The listing builds one solid part. Answer for the finished solid, in the listing's coordinates (mm). Give positions to 0.01 mm unless a question says otherwise; leave off trailing zeros. Order: outer loops, then holes, each group sorted by start corner. A loop starts at its lowest first (then second) coordinate and runs counter-clockwise, first axis right, second up. Notation, with made-up numbers: (34, 47.5) - (58, 47.5) arc R16 cw to (58, 64.5) - close; hole circle Ø3 at (-1.75, -39). An arc over 180 degrees is marked (long way). Answer in a Markdown table with one row per item.
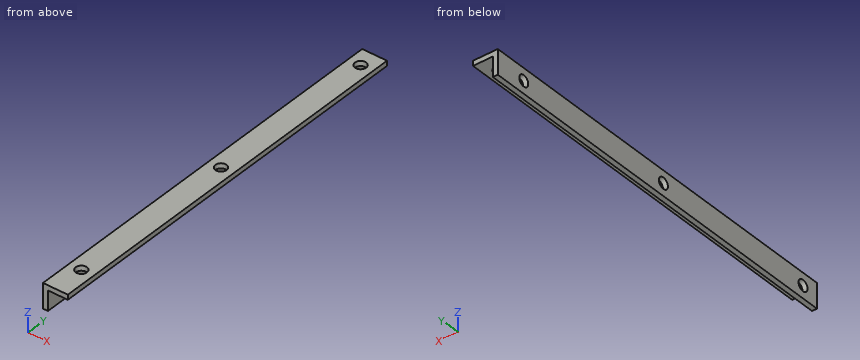
from build123d import *

# Parameters (mm, degrees)
EXTRUDE_1_DEPTH     = 160
CUT_EXTRUDE_1_REACH = 12
SKETCH_2_R          = 2.25
CUT_EXTRUDE_2_REACH = 12
SKETCH_3_R          = 2.25


with BuildPart() as part:
    # Эскиз1 → Бобышка-Вытянуть1 (new body)
    with BuildSketch(Plane(origin=(0, 0, 0), x_dir=(1, 0, 0), z_dir=(0, 1, 0))):
        Polygon((0, 10), (0, 0), (10, 0), (10, 2), (2, 2), (2, 10), align=None)
    extrude(amount=EXTRUDE_1_DEPTH)

    # Эскиз2 → Вырез-Вытянуть1 (cut, up to next)
    with BuildSketch(Plane.XY, mode=Mode.PRIVATE) as cut_extrude_1_sk1:
        with Locations((5, 13)):
            Circle(SKETCH_2_R)
    cut_extrude_1_tool1 = extrude(cut_extrude_1_sk1.sketch, amount=-CUT_EXTRUDE_1_REACH, mode=Mode.PRIVATE) & part.part
    add(cut_extrude_1_tool1.solids().sort_by_distance((5, 13, 0))[0], mode=Mode.SUBTRACT)
    # Эскиз2 → Вырез-Вытянуть1 (cut, up to next)
    with BuildSketch(Plane.XY, mode=Mode.PRIVATE) as cut_extrude_1_sk2:
        with Locations((5, 83)):
            Circle(SKETCH_2_R)
    cut_extrude_1_tool2 = extrude(cut_extrude_1_sk2.sketch, amount=-CUT_EXTRUDE_1_REACH, mode=Mode.PRIVATE) & part.part
    add(cut_extrude_1_tool2.solids().sort_by_distance((5, 83, 0))[0], mode=Mode.SUBTRACT)
    # Эскиз2 → Вырез-Вытянуть1 (cut, up to next)
    with BuildSketch(Plane.XY, mode=Mode.PRIVATE) as cut_extrude_1_sk3:
        with Locations((5, 153)):
            Circle(SKETCH_2_R)
    cut_extrude_1_tool3 = extrude(cut_extrude_1_sk3.sketch, amount=-CUT_EXTRUDE_1_REACH, mode=Mode.PRIVATE) & part.part
    add(cut_extrude_1_tool3.solids().sort_by_distance((5, 153, 0))[0], mode=Mode.SUBTRACT)

    # Эскиз3 → Вырез-Вытянуть2 (cut, up to next)
    with BuildSketch(Plane.ZY, mode=Mode.PRIVATE) as cut_extrude_2_sk1:
        with Locations((-5, 7)):
            Circle(SKETCH_3_R)
    cut_extrude_2_tool1 = extrude(cut_extrude_2_sk1.sketch, amount=-CUT_EXTRUDE_2_REACH, mode=Mode.PRIVATE) & part.part
    add(cut_extrude_2_tool1.solids().sort_by_distance((0, 7, -5))[0], mode=Mode.SUBTRACT)
    # Эскиз3 → Вырез-Вытянуть2 (cut, up to next)
    with BuildSketch(Plane.ZY, mode=Mode.PRIVATE) as cut_extrude_2_sk2:
        with Locations((-5, 77)):
            Circle(SKETCH_3_R)
    cut_extrude_2_tool2 = extrude(cut_extrude_2_sk2.sketch, amount=-CUT_EXTRUDE_2_REACH, mode=Mode.PRIVATE) & part.part
    add(cut_extrude_2_tool2.solids().sort_by_distance((0, 77, -5))[0], mode=Mode.SUBTRACT)
    # Эскиз3 → Вырез-Вытянуть2 (cut, up to next)
    with BuildSketch(Plane.ZY, mode=Mode.PRIVATE) as cut_extrude_2_sk3:
        with Locations((-5, 147)):
            Circle(SKETCH_3_R)
    cut_extrude_2_tool3 = extrude(cut_extrude_2_sk3.sketch, amount=-CUT_EXTRUDE_2_REACH, mode=Mode.PRIVATE) & part.part
    add(cut_extrude_2_tool3.solids().sort_by_distance((0, 147, -5))[0], mode=Mode.SUBTRACT)


solid = part.part
Item 1: Find section B-B on y = 153. Write down the section's boundary in (x, z), then the cut area to 3 significant figures.
Answer block:
| item | result |
|---|---|
| outline | (0, -10) - (2, -10) - (2, -2) - (2.75, -2) - (2.75, 0) - (0, 0) - close; (7.25, -2) - (10, -2) - (10, 0) - (7.25, 0) - close |
| area | 27.0 mm² |
Item 2: Find section C-C on y = 126.5. Write down the section's boundary in (x, z), then the cut area to 3 significant figures.
Answer block:
| item | result |
|---|---|
| outline | (0, -10) - (2, -10) - (2, -2) - (10, -2) - (10, 0) - (0, 0) - close |
| area | 36.0 mm² |
Item 3: Find section A-A on z = -5. Write down the section's boundary in (x, y).
Answer block:
| item | result |
|---|---|
| outline | (0, 0) - (2, 0) - (2, 4.75) - (0, 4.75) - close; (0, 9.25) - (2, 9.25) - (2, 74.75) - (0, 74.75) - close; (0, 79.25) - (2, 79.25) - (2, 144.75) - (0, 144.75) - close; (0, 149.25) - (2, 149.25) - (2, 160) - (0, 160) - close |
Item 4: Consider line 1 (Y direction, x = 5, z = -0.5); line 2 (Y direction, x = 1.6, z = -5); line 3 (Z direction, x = 0.5, y = 147). Determine where each line is inside the solid, lowest interval first.
Answer block:
| item | result |
|---|---|
| line 1 | 0 to 10.75, 15.25 to 80.75, 85.25 to 150.75, 155.25 to 160 |
| line 2 | 0 to 4.75, 9.25 to 74.75, 79.25 to 144.75, 149.25 to 160 |
| line 3 | -10 to -7.25, -2.75 to 0 |
Item 5: Each of these flat-tipped pins is pushed along its axis until it touches: P1, Ø4, axis at x = 5, y = 83.5, coming from the -Z side; P2, Ø6, axis at y = 81, z = -6, coming from the +X side; P3, Ø2.5, axis at y = 7, z = -5, coming from the -X side. Where does it stop, or does it pass through?
Answer block:
| item | result |
|---|---|
| P1 | z = -2 |
| P2 | x = 2 |
| P3 | through |
